Geometry check sheet. Reference: drawing and pictorial views, mm from the part's lowest x, y, z. A direction names the side the tool comes from. Round coordinates to 2 decimals unless told otherwise and drop trailing zeros. Write each loop counter-clockwise with the first axis right and the second up, starting at its lowest first coordinate (ties: lowest second). Pieces come first, ordered by that corner, then holes. Notation, with made-up numbers: M 88,-16 L 104,-16 A15 ccw 104,13 Z; hole C 85,11.5 d3. An arc over 180 degrees is marked long. Answer in a Markdown table with one row per item. Add a question column.
1. Sectioned sample at D-D on z = 74. Record the cut outline in (x, y), plus the area to 3 significant figures.
2. Go/stop test with flat-tipped pins: pin 1 Ø6 at (y, z) = (30.5, 15) entering from +X; pin 2 Ø12 at (x, y) = (166.5, 36) entering from +Z; pin 3 Ø10 at (y, z) = (17, 15.5) entering from -X. Record where each tip stops, or that it passes through.
3. Set-up check for the marked faces 1, 2 and 3: record each of +Z, -Z, +X, -X, +Y, -Y from which the full face is reachable in a straight line by a thin tool's end or side.
4. Sectioned sample at B-B on y = 64. Record the cut outline in (x, z).
5. Sectioned sample at C-C on x = 206. Record the cut outline in (y, z), plus the area to 3 significant figures.
6. Material ranges on probe 1 along X at (y, z) = (61, 72); probe 2 along X at (y, z) = (40, 5); probe 3 along Y at (x, z) = (20.5, 63.5), recorded low to high.
7. Sectioned sample at A-A on z = 50. Record the cut outline in (x, y), plus the area to 3 significant figures.
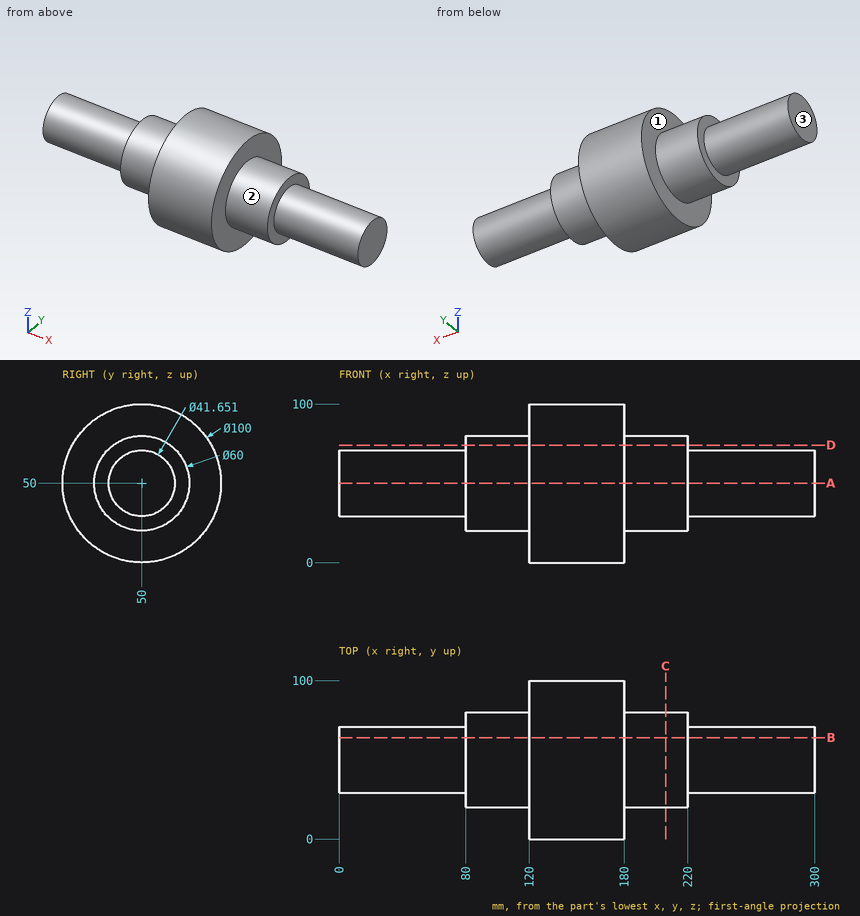
Geometry check:
| question | item | result |
|---|---|---|
| 1 | outline | M 80,32 L 120,32 L 120,6.14 L 180,6.14 L 180,32 L 220,32 L 220,68 L 180,68 L 180,93.86 L 120,93.86 L 120,68 L 80,68 Z |
| 1 | area | 8,140 mm2 |
| 2 | pin 1 | stops at x = 180 |
| 2 | pin 2 | stops at z = 99.36 |
| 2 | pin 3 | stops at x = 120 |
| 3 | face 1 | -X |
| 3 | face 2 | +X |
| 3 | face 3 | +Z, -Z, -X, +Y, -Y |
| 4 | outline | M 0,34.58 L 80,34.58 L 80,23.47 L 120,23.47 L 120,2 L 180,2 L 180,23.47 L 220,23.47 L 220,34.58 L 300,34.58 L 300,65.42 L 220,65.42 L 220,76.53 L 180,76.53 L 180,98 L 120,98 L 120,76.53 L 80,76.53 L 80,65.42 L 0,65.42 Z |
| 5 | outline | C 50,50 d60 |
| 5 | area | 2,830 mm2 |
| 6 | probe 1 | x = 80 to 220 |
| 6 | probe 2 | x = 120 to 180 |
| 6 | probe 3 | y = 34.14 to 65.86 |
| 7 | outline | M 0,29.17 L 80,29.17 L 80,20 L 120,20 L 120,0 L 180,0 L 180,20 L 220,20 L 220,29.17 L 300,29.17 L 300,70.83 L 220,70.83 L 220,80 L 180,80 L 180,100 L 120,100 L 120,80 L 80,80 L 80,70.83 L 0,70.83 Z |
| 7 | area | 17,500 mm2 |
